Design review of the part built by this model. Coordinates are the model's own, in mm. A direction names the side the tool comes from. Coordinates: 2 decimals unless noted, no trailing zeros. Loops run counter-clockwise (first coordinate to the right, second up) from the corner with the lowest first, then second, coordinate; pieces in that order, holes last. Notation, with made-up numbers: (45, 15.5) - (69, 15.5) arc R31 ccw to (69, 48.5) - close; hole circle Ø6 at (71.5, 0.25). An arc over 180 degrees is marked (long way). Answer in a Markdown table with one row per item. Add a question column.
(1) To check wall thickness, follow L1, parallel to Y at x = 17.5, z = 18.6; L2, parallel to Z at x = 2, y = -11; L3, parallel to Z at x = 5.5, y = 0. State the ranges of each line that lie inside material, in increasing order. Write a range as [from, to].
(2) For faces 1 (the face through (-15.6, 3.5, 18.6)), 2 (the face through (-1.82, -13.88, 9.42)), 3 (the face through (-15.5, -3.5, 18.6)), 4 (the face through (0, -9.5, 26)), 5 (the face through (0, -6.5, 26)), list the 3-axis set-ups (+Z, -Z, +X, -X, +Y, -Y) from which the entire face can be reached by the end or side of a thin tool; tool diameter is ignored.
(3) We need section D-D, the plane z = 8.5. Write out the cut boundary in (x, y), plus the area to 3 significant figures.
(4) We need section A-A, the plane y = 0. Write out the cut boundary in (x, z).
(5) We need section C-C, the plane y = 24.5. Write out the cut boundary in (x, z), plus the area to 3 significant figures.
(6) The part is to be moulded in two halves that separate along X. For faces 6 (the face through (-21, 0.1, 18.6)), 7 (the face through (0, -10, 23.1)), 8 (the face through (-2.72, 22.03, 15.57)), 9 (the face through (-15.497, 0.631, 18.607)), say which applies: released by +X, released by -X, zero draft, split by the parting line, or undercut.
(7) Clearance check with flat-ended pins moving along their axes: pin 1 (13.5 mm diameter, centred on x = 1, z = 8.5, fed in from +Y); pin 2 (1.9 mm diameter, centred on x = -0.5, y = 13.5, fed in from -Z); pin 3 (0.8 mm diameter, centred on x = 15.5, z = 18.5, fed in from -Y); pin 4 (1.1 mm diameter, centred on x = -16, z = 18.5, fed in from +Y). State where each tip first meets the part, or that it passes through.
(8) We need section B-B, the plane x = 0. Write out the cut boundary in (y, z).
Autodesk Inventor part; units mm, degrees
ref_plane "YZ Plane" through (0, 0, 0) normal (1, 0, 0) x (0, 1, 0)
ref_plane "XZ Plane" through (0, 0, 0) normal (0, 1, 0) x (-1, 0, 0)
ref_plane "XY Plane" through (0, 0, 0) normal (0, 0, 1) x (1, 0, 0)
sketch "スケッチ2" plane through (0, 0, 0) normal (0, 0, 1) x (1, 0, 0)
  circle A0 centre (0, 0) radius 14
  dimension "d0" = 28
extrude "本体" add sketch "スケッチ2" along normal blind 19.1
sketch "スケッチ3" plane through (0, 0, 19.1) normal (0, 0, 1) x (1, 0, 0)
  line L0 (0, 16.0197) -> (0, -16.0197) construction
  line L1 (-23.6697, 0) -> (23.6697, 0) construction
  circle A0 centre (-17.5, 0) radius 2.1
  circle A1 centre (17.5, 0) radius 2.1
  circle A2 centre (-17.5, 0) radius 3.5
  circle A3 centre (17.5, 0) radius 3.5
  line L2 (-17.5, 3.5) -> (17.5, 3.5)
  line L3 (17.5, -3.5) -> (-17.5, -3.5)
  point P0 (0, 0)
  point P1 (0, 0)
  dimension "d3" = 4.2
  dimension "d4" = 35
  dimension "d5" = 7
extrude "タブ" add sketch "スケッチ3" against normal blind 1
sketch "スケッチ4" plane through (0, 0, 19.1) normal (0, 0, 1) x (1, 0, 0)
  circle A0 centre (0, -8) radius 4.5
  point P0 (0, 0)
  dimension "d8" = 9
  dimension "d9" = 8
extrude "押し出し3" add sketch "スケッチ4" along normal blind 1.5
sketch "スケッチ5" plane through (0, -8, 20.6) normal (0, 0, 1) x (1, 0, 0)
  circle A0 centre (0, 0) radius 2.5
  circle A1 centre (0, 0) radius 4.5
  point P0 (0, 8)
  dimension "d12" = 5
extrude "押し出し4" add sketch "スケッチ5" along normal blind 2.5 contours A0
sketch "スケッチ6" plane through (0, -8, 23.1) normal (0, 0, 1) x (1, 0, 0)
  circle A0 centre (0, 0) radius 2.5
  circle A1 centre (0, 0) radius 2.5
  line L0 (-2.5, 1.5) -> (2.5, 1.5)
  line L1 (2.5, 1.5) -> (2.5, -1.5)
  line L2 (2.5, -1.5) -> (-2.5, -1.5)
  line L3 (-2.5, -1.5) -> (-2.5, 1.5)
  point P0 (0, 8)
  point P1 (2.5, 0)
  point P2 (0, 1.5)
  point P3 (-2, -1.5)
  point P4 (2, -1.5)
  point P5 (2, 1.5)
  point P6 (-2, 1.5)
  dimension "d15" = 3
extrude "押し出し5" add sketch "スケッチ6" along normal blind 6 contours A0 L2 L0
sketch "スケッチ7" plane through (0, 0, 19.1) normal (0, 0, 1) x (1, 0, 0)
  line L0 (-8.8, 0) -> (8.8, 0)
  line L1 (8.8, 0) -> (8.8, 17.1)
  line L2 (8.8, 17.1) -> (-8.8, 17.1)
  line L3 (-8.8, 17.1) -> (-8.8, 0)
  point P0 (0, 0)
  point P1 (0, 0)
  dimension "d18" = 17.6
  dimension "d19" = 17.1
extrude "押し出し6" add sketch "スケッチ7" against normal blind 16.6
sketch "スケッチ8" plane through (-8.8, 17.1, 19.1) normal (0, 1, 0) x (1, 0, 0)
  circle A0 centre (8.8, 3) radius 0.6
  line L0 (17.6, 0) -> (0, 0)
  point P0 (8.8, 19.1)
  dimension "d22" = 1.2
  dimension "d23" = 3
extrude "押し出し7" add sketch "スケッチ8" along normal blind 10
pattern_linear "矩形状パターン1" count 5 spacing 3 along (-1, 0, 0) of "押し出し7" first direction both ways yes
properties part number "28BYJ-48"
Responses:
| question | item | result |
|---|---|---|
| 1 | L1 | y = [-3.5, -2.1], [2.1, 3.5] |
| 1 | L2 | z = [0, 20.6] |
| 1 | L3 | z = [0, 19.1] |
| 2 | face 1 | +Z, -Z, -X, +Y |
| 2 | face 2 | -Z |
| 2 | face 3 | +Z, -Z, -X, -Y |
| 2 | face 4 | +Z, +X, -X, -Y |
| 2 | face 5 | +Z, +X, -X, +Y |
| 3 | outline | (-8.8, 10.89) arc R14 ccw (long way) to (8.8, 10.89) - (8.8, 17.1) - (-8.8, 17.1) - close |
| 3 | area | 688 mm2 |
| 4 | outline | (-21, 18.1) - (-19.6, 18.1) - (-19.6, 19.1) - (-21, 19.1) - close; (-15.4, 18.1) - (-14, 18.1) - (-14, 0) - (14, 0) - (14, 18.1) - (15.4, 18.1) - (15.4, 19.1) - (-15.4, 19.1) - close; (19.6, 18.1) - (21, 18.1) - (21, 19.1) - (19.6, 19.1) - close |
| 5 | outline | circle Ø1.2 at (-6, 16.1); circle Ø1.2 at (-3, 16.1); circle Ø1.2 at (0, 16.1); circle Ø1.2 at (3, 16.1); circle Ø1.2 at (6, 16.1) |
| 5 | area | 5.65 mm2 |
| 6 | face 6 | released by -X |
| 6 | face 7 | zero draft |
| 6 | face 8 | undercut |
| 6 | face 9 | undercut |
| 7 | pin 1 | stops at y = 17.1 |
| 7 | pin 2 | stops at z = 0 |
| 7 | pin 3 | stops at y = -3.5 |
| 7 | pin 4 | stops at y = 3.5 |
| 8 | outline | (-14, 0) - (14, 0) - (14, 2.5) - (17.1, 2.5) - (17.1, 15.5) - (27.1, 15.5) - (27.1, 16.7) - (17.1, 16.7) - (17.1, 19.1) - (-3.5, 19.1) - (-3.5, 20.6) - (-5.5, 20.6) - (-5.5, 23.1) - (-6.5, 23.1) - (-6.5, 29.1) - (-9.5, 29.1) - (-9.5, 23.1) - (-10.5, 23.1) - (-10.5, 20.6) - (-12.5, 20.6) - (-12.5, 19.1) - (-14, 19.1) - close |
